```python
from build123d import *

# Parameters (mm, degrees)
SKETCH1_R           = 29.21
BOSS_EXTRUDE2_DEPTH = 2.54
SKETCH2_R           = 26.67
SKETCH2_R_2         = 22.86
BOSS_EXTRUDE3_DEPTH = 5.08


with BuildPart() as part:
    # Sketch1 → Boss-Extrude2 (new body)
    with BuildSketch(Plane(origin=(0, 0, 0), x_dir=(1, 0, 0), z_dir=(0, 1, 0))):
        with Locations(Location((0, 0, 0), (0, 0, 270))):
            Circle(SKETCH1_R)
    extrude(amount=BOSS_EXTRUDE2_DEPTH)

    # Sketch2 → Boss-Extrude3 (add)
    with BuildSketch(Plane.XZ):
        with Locations(Location((0, 0, 0), (0, 0, 90))):
            Circle(SKETCH2_R)
        with Locations(Location((0, 0, 0), (0, 0, 270))):
            Circle(SKETCH2_R_2, mode=Mode.SUBTRACT)
    extrude(amount=BOSS_EXTRUDE3_DEPTH)


solid = part.part
```
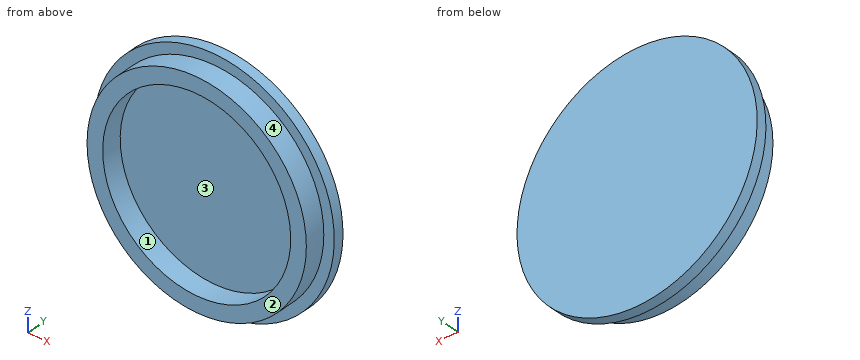
Geometry check sheet. Reference: the model listing, model coordinates, mm. Face numbers are marked on the shaded views. Round coordinates to 2 decimals unless told otherwise and drop trailing zeros. Order: outer loops, then holes, each group sorted by start corner. A loop starts at its lowest first (then second) coordinate and runs counter-clockwise, first axis right, second up. Notation, with made-up numbers: M 3,87 L 55,87 A19 ccw 55,99 Z; hole C -17,42.25 d4. An arc over 180 degrees is marked long. Answer as CSV lines item,"result".
1) Mould release check, pull along X, two halves, no side actions. Record for the marked faces 1, 2, 3 and 4: +X half, -X half, draft (parallel to the pull), parting line (faces both ways), or undercut.
Entries:
face 1,"undercut"
face 2,"draft"
face 3,"undercut"
face 4,"parting line"
2) Thickness scan on probe 1 along X at (y, z) = (-2, 0); probe 2 along X at (y, z) = (-2.75, 18); probe 3 along X at (y, z) = (0.5, 0). Record the ranges inside material, lowest first. Write a range as [from, to].
Entries:
probe 1,"[-26.67, -22.86], [22.86, 26.67]"
probe 2,"[-19.68, -14.09], [14.09, 19.68]"
probe 3,"[-29.21, 29.21]"
3) Sectioned sample at B-B on x = -4.5. Record the cut outline in (y, z), and give its area (3 significant figures).
Entries:
outline,"M -5.08,-26.29 L 0,-26.29 L 0,-28.86 L 2.54,-28.86 L 2.54,28.86 L 0,28.86 L 0,26.29 L -5.08,26.29 L -5.08,22.41 L 0,22.41 L 0,-22.41 L -5.08,-22.41 Z"
area,"186 mm2"
4) Gauge pin test, flat ends, axial feed: pin 1 Ø1 at (x, z) = (9, 19.5) entering from -Y; pin 2 Ø1 at (x, y) = (-3, -1) entering from -Z; pin 3 Ø4 at (x, y) = (-11.5, 0) entering from +Z. Record the tip position at first contact, or that the pin passes through.
Entries:
pin 1,"y = 0"
pin 2,"z = -26.55"
pin 3,"z = 27.62"
5) Sectioned sample at C-C on y = -3.25. Record the cut outline in (x, z).
Entries:
outline,"C 0,0 d53.34; hole C 0,0 d45.72"
6) Sectioned sample at A-A on z = 0. Record the cut outline in (x, y).
Entries:
outline,"M -29.21,0 L -26.67,0 L -26.67,-5.08 L -22.86,-5.08 L -22.86,0 L 22.86,0 L 22.86,-5.08 L 26.67,-5.08 L 26.67,0 L 29.21,0 L 29.21,2.54 L -29.21,2.54 Z"
